Read the model definition and answer for the solid it produces. Units are mm, in the model's axes. A direction names the side the tool comes from. Coordinates: 2 decimals unless noted, no trailing zeros. Write each loop counter-clockwise with the first axis right and the second up, starting at its lowest first coordinate (ties: lowest second). Pieces come first, ordered by that corner, then holes. Notation, with made-up numbers: (68.25, -6) -> (107.25, -6) arc R30 ccw to (107.25, 18) -> close; hole circle Ø3 at (-34.5, 75). An arc over 180 degrees is marked (long way). Use CSV: the item, a comma, the result in double quotes.
from build123d import *

# Parameters (mm, degrees)
SKETCH2_W              = 50.8
SKETCH2_H              = 76.2
BASE_FLANGE1_DEPTH     = 1.7526
SKETCHED_START         = -50.8
SKETCHED_BEND1_DEPTH   = 50.8
SKETCHED_BEND1_2_DEPTH = 50.8
CUT_EXTRUDE2_DEPTH     = 96.442377265
CUT_EXTRUDE3_REACH     = 97.512
CUT_EXTRUDE4_REACH     = 78.519
SKETCH11_R             = 3.175
CUT_EXTRUDE5_REACH     = 78.519
SKETCH12_W             = 7.62
SKETCH12_H             = 1.7145


# Read off the part's stored shape, not the designer's step: Sketched Bend1
# Sheet-metal steps are written as plain solids
with BuildPart() as part:
    # Sketch2 → Base-Flange1 (new body)
    with BuildSketch(Plane(origin=(0, 0, 0), x_dir=(0, 0, -1), z_dir=(1, 0, 0))):
        with Locations((25.4, 38.1)):
            Rectangle(SKETCH2_W, SKETCH2_H)
    extrude(amount=-BASE_FLANGE1_DEPTH)

    # Sketched Bend1 outline → Sketched Bend1 (cut)
    with BuildSketch(Plane.XY.offset(SKETCHED_START)):
        with BuildLine():
            ThreePointArc((0, 27.584427912), (-0.468104291, 25.794133277), (-1.7526, 24.462087002))
            Line((-1.7526, 24.462087002), (-1.7526, 0))
            Line((-1.7526, 0), (0, 0))
            Line((0, 0), (0, 27.584427912))
        make_face()
    extrude(amount=SKETCHED_BEND1_DEPTH, mode=Mode.SUBTRACT)

    # Sketched Bend1 2 outline → Sketched Bend1 2 (add)
    with BuildSketch(Plane.XY.offset(SKETCHED_START)):
        with BuildLine():
            ThreePointArc((-1.7526, 27.584427912), (-2.310561582, 26.237389494), (-3.6576, 25.679427912))
            Line((-3.6576, 25.679427912), (-26.873172088, 25.679427912))
            Line((-26.873172088, 25.679427912), (-26.873172088, 23.926827912))
            Line((-26.873172088, 23.926827912), (-3.6576, 23.926827912))
            ThreePointArc((-3.6576, 23.926827912), (-2.668215432, 24.063184391), (-1.7526, 24.462087002))
            Line((-1.7526, 24.462087002), (-1.7526, 27.584427912))
        make_face()
    extrude(amount=SKETCHED_BEND1_2_DEPTH)

    # Sketch9 → Cut-Extrude2 (cut, through all)
    with BuildSketch(Plane(origin=(0, 0, 0), x_dir=(0, 0, -1), z_dir=(1, 0, 0))):
        with BuildLine():
            Line((33.02, 39.751), (17.78, 39.751))
            ThreePointArc((17.78, 39.751), (6.731, 50.8), (17.78, 61.849))
            Line((17.78, 61.849), (33.02, 61.849))
            ThreePointArc((33.02, 61.849), (44.069, 50.8), (33.02, 39.751))
        make_face()
    extrude(amount=-CUT_EXTRUDE2_DEPTH, mode=Mode.SUBTRACT)

    # Sketch10 → Cut-Extrude3 (cut, up to next)
    with BuildSketch(Plane(origin=(0.2474, 0, 0), x_dir=(0, 0, -1), z_dir=(1, 0, 0)), mode=Mode.PRIVATE) as cut_extrude3_sk1:
        with BuildLine():
            Line((2.54, 68.099), (17.78, 68.099))
            ThreePointArc((17.78, 68.099), (19.53, 66.349), (17.78, 64.599))
            Line((17.78, 64.599), (2.54, 64.599))
            ThreePointArc((2.54, 64.599), (0.79, 66.349), (2.54, 68.099))
        make_face()
    cut_extrude3_tool1 = extrude(cut_extrude3_sk1.sketch, amount=-CUT_EXTRUDE3_REACH, mode=Mode.PRIVATE) & part.part
    # Sketch10 → Cut-Extrude3 (cut, up to next)
    with BuildSketch(Plane(origin=(0.2474, 0, 0), x_dir=(0, 0, -1), z_dir=(1, 0, 0)), mode=Mode.PRIVATE) as cut_extrude3_sk2:
        with BuildLine():
            Line((2.54, 33.501), (17.78, 33.501))
            ThreePointArc((17.78, 33.501), (19.53, 35.251), (17.78, 37.001))
            Line((17.78, 37.001), (2.54, 37.001))
            ThreePointArc((2.54, 37.001), (0.79, 35.251), (2.54, 33.501))
        make_face()
    cut_extrude3_tool2 = extrude(cut_extrude3_sk2.sketch, amount=-CUT_EXTRUDE3_REACH, mode=Mode.PRIVATE) & part.part
    # Sketch10 → Cut-Extrude3 (cut, up to next)
    with BuildSketch(Plane(origin=(0.2474, 0, 0), x_dir=(0, 0, -1), z_dir=(1, 0, 0)), mode=Mode.PRIVATE) as cut_extrude3_sk3:
        with BuildLine():
            Line((48.26, 33.501), (33.02, 33.501))
            ThreePointArc((33.02, 33.501), (31.27, 35.251), (33.02, 37.001))
            Line((33.02, 37.001), (48.26, 37.001))
            ThreePointArc((48.26, 37.001), (50.01, 35.251), (48.26, 33.501))
        make_face()
    cut_extrude3_tool3 = extrude(cut_extrude3_sk3.sketch, amount=-CUT_EXTRUDE3_REACH, mode=Mode.PRIVATE) & part.part
    # Sketch10 → Cut-Extrude3 (cut, up to next)
    with BuildSketch(Plane(origin=(0.2474, 0, 0), x_dir=(0, 0, -1), z_dir=(1, 0, 0)), mode=Mode.PRIVATE) as cut_extrude3_sk4:
        with BuildLine():
            Line((48.26, 68.099), (33.02, 68.099))
            ThreePointArc((33.02, 68.099), (31.27, 66.349), (33.02, 64.599))
            Line((33.02, 64.599), (48.26, 64.599))
            ThreePointArc((48.26, 64.599), (50.01, 66.349), (48.26, 68.099))
        make_face()
    cut_extrude3_tool4 = extrude(cut_extrude3_sk4.sketch, amount=-CUT_EXTRUDE3_REACH, mode=Mode.PRIVATE) & part.part
    add(cut_extrude3_tool1.solids().sort_by_distance((0.2474, 66.349, -10.16))[0], mode=Mode.SUBTRACT)
    add(cut_extrude3_tool2.solids().sort_by_distance((0.2474, 35.251, -10.16))[0], mode=Mode.SUBTRACT)
    add(cut_extrude3_tool3.solids().sort_by_distance((0.2474, 35.251, -40.64))[0], mode=Mode.SUBTRACT)
    add(cut_extrude3_tool4.solids().sort_by_distance((0.2474, 66.349, -40.64))[0], mode=Mode.SUBTRACT)

    # Sketch11 → Cut-Extrude4 (cut, up to next)
    with BuildSketch(Plane(origin=(0, 25.679427912, 0), x_dir=(1, 0, 0), z_dir=(0, 1, 0)), mode=Mode.PRIVATE) as cut_extrude4_sk1:
        with Locations(Location((-9.728172088, 38.1, 0), (0, 0, 180))):
            Circle(SKETCH11_R)
    cut_extrude4_tool1 = extrude(cut_extrude4_sk1.sketch, amount=-CUT_EXTRUDE4_REACH, mode=Mode.PRIVATE) & part.part
    add(cut_extrude4_tool1.solids().sort_by_distance((-9.728172, 25.679428, -38.1))[0], mode=Mode.SUBTRACT)

    # Sketch12 → Cut-Extrude5 (cut, up to next)
    with BuildSketch(Plane(origin=(0, 25.679427912, 0), x_dir=(1, 0, 0), z_dir=(0, 1, 0)), mode=Mode.PRIVATE) as cut_extrude5_sk1:
        with Locations((-23.063172088, 34.06775)):
            Rectangle(SKETCH12_W, SKETCH12_H)
    cut_extrude5_tool1 = extrude(cut_extrude5_sk1.sketch, amount=-CUT_EXTRUDE5_REACH, mode=Mode.PRIVATE) & part.part
    # Sketch12 → Cut-Extrude5 (cut, up to next)
    with BuildSketch(Plane(origin=(0, 25.679427912, 0), x_dir=(1, 0, 0), z_dir=(0, 1, 0)), mode=Mode.PRIVATE) as cut_extrude5_sk2:
        with Locations((-23.063172088, 42.13225)):
            Rectangle(SKETCH12_W, SKETCH12_H)
    cut_extrude5_tool2 = extrude(cut_extrude5_sk2.sketch, amount=-CUT_EXTRUDE5_REACH, mode=Mode.PRIVATE) & part.part
    add(cut_extrude5_tool1.solids().sort_by_distance((-23.063172, 25.679428, -34.06775))[0], mode=Mode.SUBTRACT)
    add(cut_extrude5_tool2.solids().sort_by_distance((-23.063172, 25.679428, -42.13225))[0], mode=Mode.SUBTRACT)


solid = part.part
1. Each of these flat-tipped pins is pushed along its axis until it touches: pin 1 Ø1.9 at (x, z) = (-1, -28) entering from -Y; pin 2 Ø4 at (x, y) = (-5, 36.5) entering from +Z; pin 3 Ø1.4 at (x, z) = (-1, -8) entering from -Y; pin 4 Ø10 at (y, z) = (35, -29.5) entering from -X. Where does it stop, or does it pass through?
Solutions:
pin 1,"stops at y = 24.35"
pin 2,"passes through"
pin 3,"stops at y = 24.49"
pin 4,"stops at x = -1.75"
2. A tool of negligible diameter and unlimited length cuts with its end or side. For faces 1 (the flat face through (-23, 25, -33.21)), 2 (the flat face through (-1, 76.2, -25)), 3 (the cylindrical face through (-0.86, 35.29, -50.01)), from which of +Z, -Z, +X, -X, +Y, -Y can it reach the whole face along a straight path? Write none if from no direction.
Solutions:
face 1,"-X, +Y, -Y"
face 2,"+Z, -Z, +X, -X, +Y"
face 3,"+X, -X"
3. A cutting plane is placed at A-A (y = 50.8). Give the vertices of the cut face in (x, z).
Solutions:
outline,"(-1.75, -50.8) -> (0, -50.8) -> (0, -44.07) -> (-1.75, -44.07) -> close; (-1.75, -6.73) -> (0, -6.73) -> (0, 0) -> (-1.75, 0) -> close"
4. Find the intervals of material crossed by line 1 along Y through (x, z) = (-8.5, -21); line 2 along X through (y, z) = (38, -42); line 3 along Z through (x, y) = (-1.5, 52.5), in increasing order.
Solutions:
line 1,"y = 23.93 to 25.68"
line 2,"x = -1.75 to 0"
line 3,"z = -50.8 to -43.94, -6.86 to 0"
5. For a pull along Y with two mould halves and no side action, classify faces 4 (the flat face through (-23, 25, -41.275)), 5 (the flat face through (-15, 25.679, -26)), 6 (the flat face through (-1, 64.599, -41)) as pulls with the +Y half, pulls with the -Y half, needs draft (parallel to the pull), parting line crosses it, or undercut.
Solutions:
face 4,"needs draft"
face 5,"pulls with the +Y half"
face 6,"undercut"
6. A cutting plane is placed at D-D (z = -38.1). Give the vertices of the cut face in (x, y) (3 decimals).
Solutions:
outline,"(-26.873, 23.927) -> (-12.903, 23.927) -> (-12.903, 25.679) -> (-26.873, 25.679) -> close; (-6.553, 23.927) -> (-3.658, 23.927) arc R3.658 ccw to (0, 27.584) -> (0, 33.501) -> (-1.753, 33.501) -> (-1.753, 27.584) arc R1.905 cw to (-3.658, 25.679) -> (-6.553, 25.679) -> close; (-1.753, 37.001) -> (0, 37.001) -> (0, 40.988) -> (-1.753, 40.988) -> close; (-1.753, 60.612) -> (0, 60.612) -> (0, 64.599) -> (-1.753, 64.599) -> close; (-1.753, 68.099) -> (0, 68.099) -> (0, 76.2) -> (-1.753, 76.2) -> close"
7. A cutting plane is placed at B-B (z = -25.5). Give the vertices of the cut face in (x, y) (3 decimals), and give its area (3 significant figures).
Solutions:
outline,"(-26.873, 23.927) -> (-3.658, 23.927) arc R3.658 ccw to (0, 27.584) -> (0, 39.751) -> (-1.753, 39.751) -> (-1.753, 27.584) arc R1.905 cw to (-3.658, 25.679) -> (-26.873, 25.679) -> close; (-1.753, 61.849) -> (0, 61.849) -> (0, 76.2) -> (-1.753, 76.2) -> close"
area,"94.8 mm^2"
8. A cutting plane is placed at C-C (x = -21.25). Give the vertices of the cut face in (y, z) (1 decimal), and give its area (3 significant figures).
Solutions:
outline,"(23.9, -50.8) -> (25.7, -50.8) -> (25.7, -43) -> (23.9, -43) -> close; (23.9, -41.3) -> (25.7, -41.3) -> (25.7, -34.9) -> (23.9, -34.9) -> close; (23.9, -33.2) -> (25.7, -33.2) -> (25.7, 0) -> (23.9, 0) -> close"
area,"83.0 mm^2"
